Can you work these out from the model? Positions are in its coordinate system, mm. A direction names the side the tool comes from. Give positions to 0.01 mm unless a question says otherwise; leave off trailing zeros. Order: outer loops, then holes, each group sorted by start corner. A loop starts at its lowest first (then second) coordinate and runs counter-clockwise, first axis right, second up. Notation, with made-up numbers: M 27,-39.5 L 81,-39.5 A21 cw 81,-11.5 Z; hole C 6.5,77 d8. An arc over 180 degrees is marked long. Use one line per item in the form item = value. Start each with the question number.
1. I want a section at B-B, the plane x = 18. List the corners of the cut face in (y, z) for me, and give its area (3 significant figures).
2. For faces 3 (the face through (5.976, -59.014, -6.524)), 4 (the face through (1, -59, 9)), 5 (the face through (5, -58, -7)), which set-ups out of +Z, -Z, +X, -X, +Y, -Y let a thin tool reach every point of the face, with its end or its side?
3. I need wall thicknesses on L1, parallel to Z at x = 0, y = -25; L2, parallel to Y at x = 4, z = 19.5; L3, parallel to X at y = -51, z = 4.5. Which ranges of each line are inside material? Lowest first, please.
4. I want a section at C-C, the plane y = -51.5. List the corners of the cut face in (x, z) for me.
5. I want a section at D-D, the plane x = 0. List the corners of the cut face in (y, z) for me (3 decimals), and give its area (3 significant figures).
6. We'd pull the mould along X, two halves only. Please class faces 1 (the face through (-23.255, 3.131, -14.281)), 2 (the face through (6, 0, 14)): +X half, -X half, draft (parallel to the pull), parting line (faces both ways), or undercut.
7. I want a section at A-A, the plane z = 0. List the corners of the cut face in (x, y) for me (3 decimals), and give its area (3 significant figures).
8. Will these pins go through, and if not, where does the flat tip stop? P1, Ø1, axis at x = -5.5, z = -7, coming from the -Y side; P2, Ø2, axis at x = -7.5, z = 22, coming from the -Y side; P3, Ø4, axis at y = -11.5, z = -11.5, coming from the -X side; P4, Ø5, axis at x = -17, y = -7.5, coming from the +Z side.
```python
from build123d import *

# Parameters (mm, degrees)
SKETCH5_R                   = 7.5
CUT_EXTRUDE1_DEPTH          = 90
SKETCH6_R                   = 3.5
CUT_EXTRUDE2_DEPTH          = 20
CIRPATTERN1_COUNT           = 6
SKETCH11_R                  = 3.18
CUT_EXTRUDE4_DEPTH          = 101.105860558
SKETCH23_R                  = 30.48
CUT_EXTRUDE6_DEPTH          = 80.122584091
F_1_4_CLEARANCE_HOLE1_D     = 6.5278
F_1_4_CLEARANCE_HOLE1_DEPTH = 15.4203
F_1_4_CLEARANCE_HOLE1_TIP   = 1.961148974
CHAMFER1_SIZE               = 3.175
SKETCH26_OUTSIDE_W          = 84.718
SKETCH26_OUTSIDE_H          = 84.718
SKETCH26_OUTSIDE_R          = 15
FOR_TURNING_EASE_DEPTH      = 74.878689756
SKETCH29_W                  = 2
SKETCH29_H                  = 2
CUT_EXTRUDE7_DEPTH          = 74.878689756
CIRPATTERN4_COUNT           = 5


with BuildPart() as part:
    # Sketch1 → Revolve1 (revolve)
    with BuildSketch(Plane(origin=(0, 0, 0), x_dir=(0, 0, -1), z_dir=(1, 0, 0))):
        Polygon((0, 30.35), (12.7, 30.35), (12.7, 6.35), (30.48, 6.35), (30.48, 0), (15.68, 0), (10.16, -20.600920458), (10.16, -60), (0, -60), align=None)
    revolve(axis=Axis((0, 0, 0), (0, 1, 0)))

    # Sketch5 → Cut-Extrude1 (cut)
    with BuildSketch(Plane.XZ.offset(60)):
        with Locations(Location((0, 0, 0), (0, 0, 270))):
            Circle(SKETCH5_R)
    extrude(amount=-CUT_EXTRUDE1_DEPTH, mode=Mode.SUBTRACT)

    # Sketch6 → Cut-Extrude2 (cut, symmetric)
    with BuildSketch(Plane.XY):
        with Locations((0, 16.659966967)):
            Circle(SKETCH6_R)
    cut_extrude2 = extrude(amount=CUT_EXTRUDE2_DEPTH, both=True, mode=Mode.SUBTRACT)

    # CirPattern1: Cut-Extrude2 ×6 about axis
    cirpattern1_axis = Axis((0, 30.35, 0), (0, -1, 0))
    for i in range(1, CIRPATTERN1_COUNT):
        add(cut_extrude2.rotate(cirpattern1_axis, i * 360 / CIRPATTERN1_COUNT), mode=Mode.SUBTRACT)

    # Sketch11 → Cut-Extrude4 (cut, through all)
    with BuildSketch(Plane(origin=(0, 30.35, 0), x_dir=(1, 0, 0), z_dir=(0, 1, 0))):
        with Locations(Location((0, 0, 0), (0, 0, 270))):
            Circle(SKETCH11_R)
    extrude(amount=-CUT_EXTRUDE4_DEPTH, mode=Mode.SUBTRACT)

    # Sketch23 → Cut-Extrude6 (cut, through all)
    with BuildSketch(Plane(origin=(0, 6.35, 0), x_dir=(1, 0, 0), z_dir=(0, 1, 0))):
        with Locations(Location((0, 0, 0), (0, 0, 90))):
            Circle(SKETCH23_R)
    extrude(amount=CUT_EXTRUDE6_DEPTH, mode=Mode.SUBTRACT)

    # 1_4 Clearance Hole1
    with Locations(Plane(origin=(0, 6.35, 0), x_dir=(1, 0, 0), z_dir=(0, 1, 0))):
        with Locations((-20.240427094, 15.531025958), (23.570476573, 9.763211068), (20.240427094, -15.531025958), (-23.570476573, -9.763211068)):
            Hole(F_1_4_CLEARANCE_HOLE1_D / 2, depth=F_1_4_CLEARANCE_HOLE1_DEPTH)
            with Locations((0, 0, -(F_1_4_CLEARANCE_HOLE1_DEPTH + F_1_4_CLEARANCE_HOLE1_TIP / 2))):  # 118° drill point
                Cone(0, F_1_4_CLEARANCE_HOLE1_D / 2, F_1_4_CLEARANCE_HOLE1_TIP, mode=Mode.SUBTRACT)

    # Chamfer1
    chamfer1_edges = [part.edges().sort_by_distance(p)[0] for p in [
        (0, 6.35, 7.5),
    ]]
    chamfer(chamfer1_edges, length=CHAMFER1_SIZE)

    # Sketch26 outside → for-turning-ease (cut, through all)
    with BuildSketch(Plane.XZ):
        Rectangle(SKETCH26_OUTSIDE_W, SKETCH26_OUTSIDE_H)
        with Locations(Location((0, 0, 0), (0, 0, 90))):
            Circle(SKETCH26_OUTSIDE_R, mode=Mode.SUBTRACT)
    extrude(amount=FOR_TURNING_EASE_DEPTH, mode=Mode.SUBTRACT)

    # Sketch29 → Cut-Extrude7 (cut, symmetric)
    with BuildSketch(Plane.XY):
        with Locations((0, -59)):
            Rectangle(SKETCH29_W, SKETCH29_H)
    cut_extrude7 = extrude(amount=CUT_EXTRUDE7_DEPTH, both=True, mode=Mode.SUBTRACT)

    # CirPattern4: Cut-Extrude7 ×5 about axis
    cirpattern4_axis = Axis((0, 0, 0), (0, 1, 0))
    for i in range(1, CIRPATTERN4_COUNT):
        add(cut_extrude7.rotate(cirpattern4_axis, i * 360 / CIRPATTERN4_COUNT), mode=Mode.SUBTRACT)


solid = part.part
```
Check result:
q1.outline = M 0,-24.6 L 6.35,-24.6 L 6.35,13.16 L 0,13.16 Z; M 0,17.9 L 6.35,17.9 L 6.35,24.6 L 0,24.6 Z
q1.area = 282 mm2
q2.face_3 = -Z, -Y
q2.face_4 = +Z, -Z, -Y
q2.face_5 = -Y
q3.L1 = -10.16 to -7.5, 7.5 to 10.16
q3.L2 = 0 to 6.35
q3.L3 = -9.11 to -6, 6 to 9.11
q4.outline = C 0,0 d20.32; hole C 0,0 d15
q5.outline = M -58,-10.16 L -20.601,-10.16 L -2.538,-15 L 0,-15 L 0,-30.48 L 6.35,-30.48 L 6.35,-10.675 L 3.175,-7.5 L -58,-7.5 Z; M -58,7.5 L 3.175,7.5 L 6.35,10.675 L 6.35,30.48 L 0,30.48 L 0,15 L -2.538,15 L -20.601,10.16 L -58,10.16 Z
q5.area = 702 mm2
q6.face_1 = undercut
q6.face_2 = draft
q7.outline = M -30.48,0 L -15,0 L -15,-2.538 L -10.16,-20.601 L -10.16,-60 L -7.5,-60 L -7.5,3.175 L -10.675,6.35 L -30.48,6.35 Z; M 7.5,-60 L 10.16,-60 L 10.16,-20.601 L 15,-2.538 L 15,0 L 30.48,0 L 30.48,6.35 L 10.675,6.35 L 7.5,3.175 Z
q7.area = 713 mm2
q8.P1 = -58
q8.P2 = 0
q8.P3 = -8.42
q8.P4 = through
